Part model, mm, in its own coordinate system. A direction names the side the tool comes from. Round coordinates to 2 decimals unless told otherwise and drop trailing zeros. Loops run counter-clockwise (first coordinate to the right, second up) from the corner with the lowest first, then second, coordinate; pieces in that order, holes last.
1) Band-saw the part on A-A, the plane x = 10. Write the cut outline in (y, z).
2) Band-saw the part on B-B, the plane z = -46. Write the cut outline in (x, y).
3) Band-saw the part on D-D, the plane z = -38. Write the cut outline in (x, y).
4) 3-axis set-ups, long thin cutter, end or side, ignore diameter. For faces 1 (the flat face through (30, 0, -15)), 2 (the flat face through (48, 5, -13)), 3 (the cylindrical face through (51.69, 2.46, -16.84)): which of +Z, -Z, +X, -X, +Y, -Y reach the whole face in a straight line?
5) Band-saw the part on C-C, the plane y = 9.75. Write the cut outline in (x, z), then the cut area to 3 significant figures.
6) Mould opens along X. For faces 4 (the flat face through (47.5, 7, -43)), 5 (the flat face through (11.5, 5, -12.7)), 6 (the flat face through (0, 10, -28)), 7 (the flat face through (54, 7, -55)) say: +X half, -X half, draft (parallel to the pull), parting line (faces both ways), or undercut.
7) Drop flat-ended pins along their axis: P1, Ø4.5, axis at x = 10, z = -15, coming from the -Y side; P2, Ø6.5, axis at x = 50, z = -15, coming from the +Y side; P3, Ø2, axis at x = 50, y = 17.5, coming from the +Z side; P4, Ø12, axis at x = 39, z = -16, coming from the -Y side. Give the stop position or say it passes through.
8) Probe line 1 (X direction, y = 3.45, z = -15); line 2 (Y direction, x = 9.25, z = -46); line 3 (X direction, y = 8.5, z = -41). List the from-to ranges inside material, lowest first.
from build123d import *

# Parameters (mm, degrees)
CROQUIS1_R                   = 2.5
SALIENTE_EXTRUIR1_DEPTH      = 5
SALIENTE_EXTRUIR2_DEPTH      = 15
SALIENTE_EXTRUIR2_DEPTH_BACK = 10
CORTAR_EXTRUIR2_REACH        = 85.815
CROQUIS4_R                   = 3.1
CROQUIS4_W                   = 30
CROQUIS4_H                   = 5
REDONDEO2_R                  = 7
CORTAR_EXTRUIR3_DEPTH        = 10
CORTAR_EXTRUIR3_DEPTH_BACK   = 10
CROQUIS5_R                   = 5.5


with BuildPart() as part:
    # Croquis1 → Saliente-Extruir1 (new body)
    with BuildSketch(Plane(origin=(0, 0, 0), x_dir=(1, 0, 0), z_dir=(0, 1, 0))):
        Polygon((0, 0), (60, 0), (60, 30), (60, 55), (47.5, 55), (47.5, 30), (12.5, 30), (12.5, 55), (0, 55), (0, 30), align=None)
        with Locations(Location((10, 15, 0), (0, 0, 270))):
            Circle(CROQUIS1_R, mode=Mode.SUBTRACT)
        with Locations(Location((50, 15, 0), (0, 0, 270))):
            Circle(CROQUIS1_R, mode=Mode.SUBTRACT)
    extrude(amount=SALIENTE_EXTRUIR1_DEPTH)

    # Croquis2 → Saliente-Extruir2 (add, two sides: drawn at the far end of the back side and taken through both)
    with BuildSketch(Plane(origin=(0, 5, 0), x_dir=(1, 0, 0), z_dir=(0, 1, 0)).offset(-SALIENTE_EXTRUIR2_DEPTH_BACK)):
        Polygon((3, 0), (3, 25), (17, 25), (17, 0), (43, 0), (43, 25), (57, 25), (57, 0), (60, 0), (60, 55), (47.5, 55), (47.5, 30), (12.5, 30), (12.5, 55), (0, 55), (0, 0), align=None)
    extrude(amount=SALIENTE_EXTRUIR2_DEPTH + SALIENTE_EXTRUIR2_DEPTH_BACK)

    # Cortar-Extruir2: up to this face of the body (flat: up to its plane)
    cortar_extruir2_end = Plane(part.part.faces().sort_by_distance((60, 7.5, -27.5))[0])
    # Croquis4 → Cortar-Extruir2 (cut, up to the picked face)
    with BuildSketch(Plane.ZY, mode=Mode.PRIVATE) as cortar_extruir2_sk1:
        with Locations((-46, 12)):
            Circle(CROQUIS4_R)
    cortar_extruir2_tool1 = split(extrude(cortar_extruir2_sk1.sketch, amount=-CORTAR_EXTRUIR2_REACH, mode=Mode.PRIVATE), bisect_by=cortar_extruir2_end, keep=Keep.BOTH, mode=Mode.PRIVATE)
    # Croquis4 → Cortar-Extruir2 (cut, up to the picked face)
    with BuildSketch(Plane.ZY, mode=Mode.PRIVATE) as cortar_extruir2_sk2:
        with Locations((-15, -2.5)):
            Rectangle(CROQUIS4_W, CROQUIS4_H)
    cortar_extruir2_tool2 = split(extrude(cortar_extruir2_sk2.sketch, amount=-CORTAR_EXTRUIR2_REACH, mode=Mode.PRIVATE), bisect_by=cortar_extruir2_end, keep=Keep.BOTH, mode=Mode.PRIVATE)
    add(cortar_extruir2_tool1.solids().sort_by(Axis((0, 12, -46), (1, 0, 0)))[0], mode=Mode.SUBTRACT)
    add(cortar_extruir2_tool2.solids().sort_by(Axis((0, -2.5, -15), (1, 0, 0)))[0], mode=Mode.SUBTRACT)

    # Redondeo2
    redondeo2_edges = [part.edges().sort_by_distance(p)[0] for p in [
        (6.25, -5, -55),
        (53.75, -5, -55),
        (6.25, 20, -55),
        (1.5, 20, 0),
        (30, 20, 0),
        (58.5, 20, 0),
        (53.75, 20, -55),
    ]]
    fillet(redondeo2_edges, radius=REDONDEO2_R)

    # Croquis5 → Cortar-Extruir3 (cut, two sides: drawn at the far end of the back side and taken through both)
    with BuildSketch(Plane(origin=(0, -5, -5), x_dir=(-1, 0, 0), z_dir=(0, -0.7071067811865488, -0.7071067811865464)).offset(-CORTAR_EXTRUIR3_DEPTH_BACK)):
        with Locations((-30, 35.355339059)):
            Circle(CROQUIS5_R)
    extrude(amount=CORTAR_EXTRUIR3_DEPTH + CORTAR_EXTRUIR3_DEPTH_BACK, mode=Mode.SUBTRACT)


solid = part.part
Reported:
1. outline: (-5, -48) arc R7 ccw to (2, -55) - (13, -55) arc R7 ccw to (20, -48) - (20, -25) - (5, -25) - (5, -17.5) - (0, -17.5) - (0, -30) - (-5, -30) - close; (0, -12.5) - (5, -12.5) - (5, 0) - (0, 0) - close; hole circle Ø6.2 at (12, -46)
2. outline: (0, -5) - (12.5, -5) - (12.5, 8.9) - (0, 8.9) - close; (0, 15.1) - (12.5, 15.1) - (12.5, 20) - (0, 20) - close; (47.5, -5) - (60, -5) - (60, 8.9) - (47.5, 8.9) - close; (47.5, 15.1) - (60, 15.1) - (60, 20) - (47.5, 20) - close
3. outline: (0, -5) - (12.5, -5) - (12.5, 20) - (0, 20) - close; (47.5, -5) - (60, -5) - (60, 20) - (47.5, 20) - close
4. face 1: +Z, +X, -X, -Y
4. face 2: +Z, +Y
4. face 3: +Y, -Y
5. outline: (0, -55) - (12.5, -55) - (12.5, -48.13) - (0, -48.13) - close; (0, -43.87) - (12.5, -43.87) - (12.5, -30) - (47.5, -30) - (47.5, -43.87) - (60, -43.87) - (60, 0) - (57, 0) - (57, -25) - (43, -25) - (43, 0) - (17, 0) - (17, -25) - (3, -25) - (3, 0) - (0, 0) - close; (47.5, -55) - (60, -55) - (60, -48.13) - (47.5, -48.13) - close
5. area: 1,620 mm2
6. face 4: undercut
6. face 5: undercut
6. face 6: -X half
6. face 7: draft
7. P1: passes through
7. P2: stops at y = 5
7. P3: stops at z = -25
7. P4: stops at y = 0
8. line 1: x = 0 to 7.5, 12.5 to 47.5, 52.5 to 60
8. line 2: y = -5 to 8.9, 15.1 to 20
8. line 3: x = 0 to 12.5, 47.5 to 60
